Input: dimensioned drawing with shaded views. Units: mm. Origin: part minimum x, y, z. Round coordinates to 2 decimals unless told otherwise and drop trailing zeros. Order: outer loops, then holes, each group sorted by start corner. A loop starts at its lowest first (then second) coordinate and runs counter-clockwise, first axis right, second up. Notation, with made-up numbers: M 86.25,42.5 L 133.25,42.5 A23 cw 133.25,50.5 Z; hole C -35,83 d2. An arc over 180 degrees is marked long. Answer as CSV lines item,"result". Start each with the question number.
Item 1: First-contact query: P1, Ø9, axis at x = 256.5, z = 4.5, coming from the -Y side; P2, Ø3, axis at x = 177, y = 140.5, coming from the -Z side; P3, Ø4, axis at x = 166.5, y = 42, coming from the +Z side; P4, Ø6.5, axis at x = 14.5, z = 3.5, coming from the +Y side. Flat tips, straight axial feed; report the tip coordinate or a pass-through.
Item 2: Section query B-B on y = 82. Return the cut outline in (x, z), plus the area to 3 significant figures.
Item 3: Line query: line 1 (X direction, y = 105.5, z = 5.5); line 2 (Y direction, x = 53, z = 4.75); line 3 (Z direction, x = 23, y = 130). Output: solid intervals per line, ascending. Write a range as [from, to].
Item 4: Section query D-D on x = 185. Return the cut outline in (y, z), plus the area to 3 significant figures.
Item 5: Section query A-A on x = 35. Return the cut outline in (y, z), plus the area to 3 significant figures.
Item 6: Section query C-C on y = 10. Return the cut outline in (x, z), plus the area to 3 significant figures.
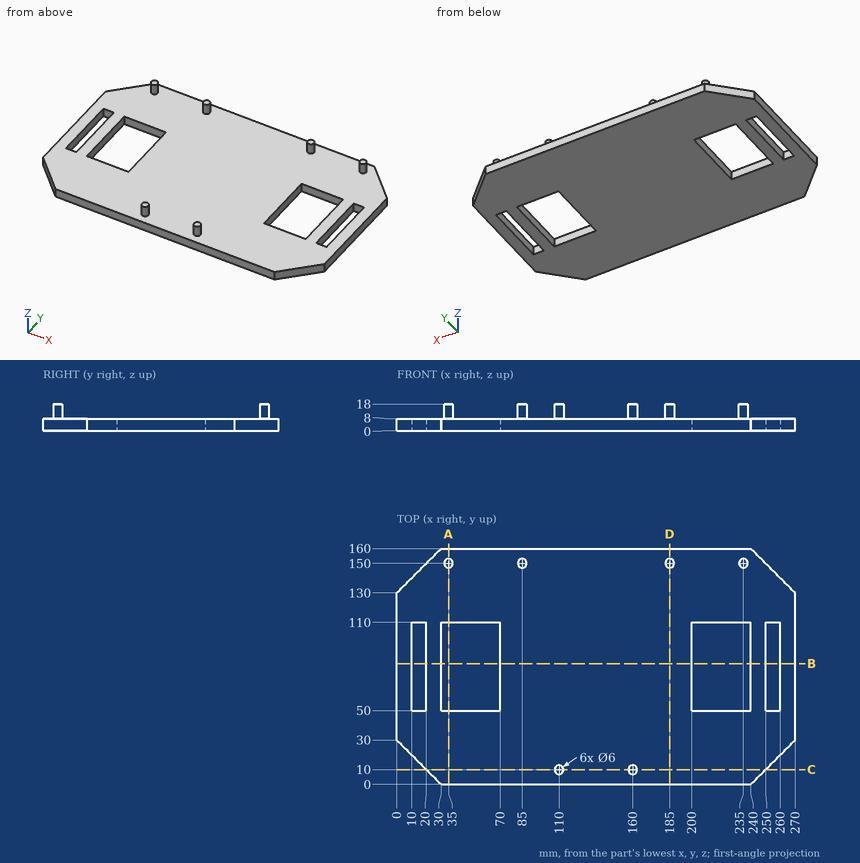
Results:
1,P1,"y = 12"
1,P2,"z = 0"
1,P3,"z = 8"
1,P4,"y = 147.75"
2,outline,"M 0,0 L 10,0 L 10,8 L 0,8 Z; M 20,0 L 30,0 L 30,8 L 20,8 Z; M 70,0 L 200,0 L 200,8 L 70,8 Z; M 240,0 L 250,0 L 250,8 L 240,8 Z; M 260,0 L 270,0 L 270,8 L 260,8 Z"
2,area,"1,360 mm^2"
3,line 1,"[0, 10], [20, 30], [70, 200], [240, 250], [260, 270]"
3,line 2,"[0, 50], [110, 160]"
3,line 3,"[0, 8]"
4,outline,"M 0,0 L 160,0 L 160,8 L 153,8 L 153,18 L 147,18 L 147,8 L 0,8 Z"
4,area,"1,340 mm^2"
5,outline,"M 0,0 L 50,0 L 50,8 L 0,8 Z; M 110,0 L 160,0 L 160,8 L 153,8 L 153,18 L 147,18 L 147,8 L 110,8 Z"
5,area,"860 mm^2"
6,outline,"M 20,0 L 250,0 L 250,8 L 163,8 L 163,18 L 157,18 L 157,8 L 113,8 L 113,18 L 107,18 L 107,8 L 20,8 Z"
6,area,"1,960 mm^2"
